```python
from build123d import *

# Parameters (mm, degrees)
BOSS_EXTRUDE1_DEPTH         = 14
BOSS_EXTRUDE1_DEPTH_BACK    = 14
SKETCH1_R                   = 4
CUT_EXTRUDE_THIN9_START     = -12
CUT_EXTRUDE_THIN9_OUTLINE_R = 4
CUT_EXTRUDE_THIN9_DEPTH     = 24


# Read off the part's stored shape, not the designer's step: Cut-Extrude-Thin9
with BuildPart() as part:
    # Sketch1 → Boss-Extrude1 (new, two sides: drawn at the far end of the back side and taken through both)
    with BuildSketch(Plane.XY.offset(-BOSS_EXTRUDE1_DEPTH_BACK)):
        with BuildLine():
            ThreePointArc((-17.839605582, 6.651694239), (-34.292375842, -0.987792391), (-17.839605582, -8.627279021))
            Line((-17.839605582, -8.627279021), (19.254853898, -8.627279021))
            ThreePointArc((19.254853898, -8.627279021), (35.707624158, -0.987792391), (19.254853898, 6.651694239))
            Line((19.254853898, 6.651694239), (-17.839605582, 6.651694239))
        make_face()
        with Locations((-24.292375842, -0.987792391)):
            Circle(SKETCH1_R, mode=Mode.SUBTRACT)
        with Locations((25.707624158, -0.987792391)):
            Circle(SKETCH1_R, mode=Mode.SUBTRACT)
    extrude(amount=BOSS_EXTRUDE1_DEPTH + BOSS_EXTRUDE1_DEPTH_BACK)

    # Cut-Extrude-Thin9 outline → Cut-Extrude-Thin9 (cut)
    # profile 1 of 2: a face of its own
    with BuildSketch(Plane.XY.offset(CUT_EXTRUDE_THIN9_START)):
        with BuildLine():
            ThreePointArc((13.975691494, 6.651694239), (11.707624158, -0.987792391), (13.975691494, -8.627279021))
            Line((13.975691494, -8.627279021), (19.254853898, -8.627279021))
            ThreePointArc((19.254853898, -8.627279021), (35.707624158, -0.987792391), (19.254853898, 6.651694239))
            Line((19.254853898, 6.651694239), (13.975691494, 6.651694239))
        make_face()
        with Locations((25.707624158, -0.987792391)):
            Circle(CUT_EXTRUDE_THIN9_OUTLINE_R, mode=Mode.SUBTRACT)
    # profile 2 of 2: a face of its own
    with BuildSketch(Plane.XY.offset(CUT_EXTRUDE_THIN9_START)):
        with BuildLine():
            Line((-17.839605582, -8.627279021), (-12.560443178, -8.627279021))
            ThreePointArc((-12.560443178, -8.627279021), (-10.292375842, -0.987792391), (-12.560443178, 6.651694239))
            Line((-12.560443178, 6.651694239), (-17.839605582, 6.651694239))
            ThreePointArc((-17.839605582, 6.651694239), (-34.292375842, -0.987792391), (-17.839605582, -8.627279021))
        make_face()
        with Locations((-24.292375842, -0.987792391)):
            Circle(CUT_EXTRUDE_THIN9_OUTLINE_R, mode=Mode.SUBTRACT)
    extrude(amount=CUT_EXTRUDE_THIN9_DEPTH, mode=Mode.SUBTRACT)


solid = part.part
```
The listing builds one solid part. Answer for the finished solid, in the listing's coordinates (mm). A direction names the side the tool comes from. Round coordinates to 2 decimals unless told otherwise and drop trailing zeros. Order: outer loops, then holes, each group sorted by start corner. A loop starts at its lowest first (then second) coordinate and runs counter-clockwise, first axis right, second up. Notation, with made-up numbers: (-28, 28) -> (-20, 28) arc R21 cw to (-20, 50) -> close; hole circle Ø9 at (31, -27.75). An arc over 180 degrees is marked (long way). Answer as CSV lines item,"result". Start each with the question number.
(1) Flat-ended cylindrical pins translate along their axes: pin 1 Ø4 at (y, z) = (-1, 6) entering from +X; pin 2 Ø10.5 at (x, y) = (25.71, -0.99) entering from -Z; pin 3 Ø2 at (x, z) = (9.5, 3.5) entering from -Y; pin 4 Ø8.5 at (x, z) = (-8.5, -4) entering from +Y. Find the tip coordinate at first contact, or state that the pin passes through.
(2) Find the intervals of material crossed by probe 1 along Z at (x, y) = (29.5, 1.5); probe 2 along X at (y, z) = (-2.75, 12.75); probe 3 along Y at (x, z) = (1.5, 9), in increasing order. Write a range as from..to.
(3) For a pull along Z with two mould halves and no side action, classify faces 6 (the face through (-34.287, -0.67, 12.986)), 7 (the face through (0, -1, 14)), 8 (the face through (-10.293, -1.101, -0.168)) as +Z half, -Z half, draft (parallel to the pull), parting line (faces both ways), or undercut.
(4) The part is cut by section B-B (y = -2.25). Determine the outline of the cut face in (x, z).
(5) The part is cut by section C-C (y = 7.75). Determine the outline of the cut face in (x, z).
(6) The part is cut by section A-A (x = -17). Determine the outline of the cut face in (y, z).
(7) The part is cut by section D-D (x = 26). Determine the outline of the cut face in (y, z).
(8) A tool of negligible diameter and unlimited length cuts with its end or side. For faces 1 (the face through (0, -8.627, 0)), 2 (the face through (0, -1, -14)), 3 (the face through (-34.287, -0.67, -13.014)), 4 (the face through (11.71, -0.87, -0.17)), 5 (the face through (1, 6.652, 0)), from which of +Z, -Z, +X, -X, +Y, -Y can it reach the whole face along a straight path? Write none if from no direction.
Evaluation:
1,pin 1,"x = 11.85"
1,pin 2,"z = -14"
1,pin 3,"y = -8.63"
1,pin 4,"y = 6.65"
2,probe 1,"-14..-12, 12..14"
2,probe 2,"-34.14..-27.88, -20.7..22.12, 29.3..35.55"
2,probe 3,"-8.63..6.65"
3,face 6,"draft"
3,face 7,"+Z half"
3,face 8,"undercut"
4,outline,"(-34.21, -14) -> (-28.09, -14) -> (-28.09, -12) -> (-34.21, -12) -> close; (-34.21, 12) -> (-28.09, 12) -> (-28.09, 14) -> (-34.21, 14) -> close; (-20.5, -14) -> (21.91, -14) -> (21.91, -12) -> (11.76, -12) -> (11.76, 12) -> (21.91, 12) -> (21.91, 14) -> (-20.5, 14) -> (-20.5, 12) -> (-10.35, 12) -> (-10.35, -12) -> (-20.5, -12) -> close; (29.5, -14) -> (35.63, -14) -> (35.63, -12) -> (29.5, -12) -> close; (29.5, 12) -> (35.63, 12) -> (35.63, 14) -> (29.5, 14) -> close"
5,outline,"(-29.16, -14) -> (-19.43, -14) -> (-19.43, -12) -> (-29.16, -12) -> close; (-29.16, 12) -> (-19.43, 12) -> (-19.43, 14) -> (-29.16, 14) -> close; (20.84, -14) -> (30.57, -14) -> (30.57, -12) -> (20.84, -12) -> close; (20.84, 12) -> (30.57, 12) -> (30.57, 14) -> (20.84, 14) -> close"
6,outline,"(-8.63, -14) -> (6.65, -14) -> (6.65, -12) -> (-8.63, -12) -> close; (-8.63, 12) -> (6.65, 12) -> (6.65, 14) -> (-8.63, 14) -> close"
7,outline,"(-10.98, -14) -> (-4.98, -14) -> (-4.98, -12) -> (-10.98, -12) -> close; (-10.98, 12) -> (-4.98, 12) -> (-4.98, 14) -> (-10.98, 14) -> close; (3, -14) -> (9.01, -14) -> (9.01, -12) -> (3, -12) -> close; (3, 12) -> (9.01, 12) -> (9.01, 14) -> (3, 14) -> close"
8,face 1,"+Z, -Z, -Y"
8,face 2,"-Z, +X, -X, +Y, -Y"
8,face 3,"+Z, -Z"
8,face 4,"+X"
8,face 5,"+Z, -Z, +Y"
